Geometry check sheet. Reference: the model listing, model coordinates, mm. A direction names the side the tool comes from. Round coordinates to 2 decimals unless told otherwise and drop trailing zeros. Write each loop counter-clockwise with the first axis right and the second up, starting at its lowest first coordinate (ties: lowest second). Pieces come first, ordered by that corner, then holes. Notation, with made-up numbers: M 32.25,45.5 L 76.25,45.5 A34 ccw 76.25,81.5 Z; hole C 75,-12 d5. An arc over 180 degrees is marked long. One line per item, written item: value. Start each with the question number.
1. Section check D-D (x = 1.75). Count the separate pieces of the cut face and the enclosed holes in it, and give its area (3 significant figures).
2. Access from +Z, -Z, +X, -X, +Y, -Y to the whole of each face (thin tool, end or side, straight path). Record for faces 4 (the cylindrical face through (-10.5, 3.5, 0)), 5 (the flat face through (0, 3, -15)), 6 (the flat face through (7.5, 10, -19)), 7 (the flat face through (5, 15, -15)), 8 (the flat face through (-7.5, 10, -19)).
3. Section check C-C (z = -18.5). Record the boundary of the cut face in (x, y).
4. Release check for a two-part mould opening along Y. For faces 1 (the flat face through (3, 7, -3)), 2 (the flat face through (-0.5, 4, 9)), 3 (the cylindrical face through (2.72, 4.22, 18.77)) record: pulls with the +Y half, pulls with the -Y half, needs draft (parallel to the pull), parting line crosses it, or undercut.
5. Section check A-A (x = 6.5). Record the boundary of the cut face in (y, z).
6. Section check B-B (y = 15). Record the boundary of the cut face in (x, z), and give its area (3 significant figures).
7. Scan lines: probe 1 along Y at (x, z) = (-4.6, -18.5); probe 2 along X at (y, z) = (3, -16); probe 3 along Y at (x, z) = (-1.55, 16.5). Record each from-to range of solid material in increasing order. Write a range as [from, to].
8. Depth check by flat-ended pin: P1, Ø3.5, axis at y = 3.5, z = 16, coming from the -X side; P2, Ø5.5, axis at y = 3.5, z = 16.5, coming from the +X side; P3, Ø5.5, axis at x = 5, y = 16, coming from the +Z side; P4, Ø4, axis at y = 5, z = -18.5, coming from the +X side. Enter the tip coordinate at first touch or a pass-through.
from build123d import *

# Parameters (mm, degrees)
SKETCH1_W           = 5
SKETCH1_H           = 7
BOSS_EXTRUDE1_DEPTH = 7
SKETCH3_R           = 2.38125
CUT_EXTRUDE2_DEPTH  = 29.969811874
FILLET2_R           = 3.5
SKETCH5_W           = 1
SKETCH5_H           = 8.5
CUT_EXTRUDE4_DEPTH  = 27.253571186
SKETCH6_R           = 1.5
CUT_EXTRUDE5_DEPTH  = 27.253571186
SKETCH8_W           = 5
SKETCH8_H           = 7
BOSS_EXTRUDE2_DEPTH = 13
FILLET3_DEPTH       = 20
FILLET3_2_DEPTH     = 8.22694
FILLET3_START       = -9.48212727
FILLET3_3_DEPTH     = 6.98212727
FILLET3_START_2     = 2.5
FILLET3_4_DEPTH     = 6.98212727
FILLET3_START_3     = 7
FILLET3_5_DEPTH     = 13.0000001
CHAMFER1_SIZE       = 2.5
CHAMFER2_SIZE       = 1
SKETCH9_R           = 1.5
CUT_EXTRUDE7_DEPTH  = 36.832945734


with BuildPart() as part:
    # Sketch1 → Boss-Extrude1 (new body)
    with BuildSketch(Plane(origin=(0, 0, 0), x_dir=(1, 0, 0), z_dir=(0, 1, 0))):
        with BuildLine():
            Line((-5, -5), (-5, -11.456439237))
            ThreePointArc((-5, -11.456439237), (0, -12.5), (5, -11.456439237))
            Line((5, -11.456439237), (5, -5))
            Line((5, -5), (-5, -5))
        make_face()
        with BuildLine():
            ThreePointArc((-11.620226592, 4.606553371), (-11.556942324, -4.763096065), (-5, -11.456439237))
            Line((-5, -11.456439237), (-5, -5))
            Line((-5, -5), (5, -5))
            Line((5, -5), (5, -11.456439237))
            ThreePointArc((5, -11.456439237), (10.458250332, -6.846531969), (12.5, 0))
            ThreePointArc((12.5, 0), (12.27808683, 2.344905926), (11.620226592, 4.606553371))
            ThreePointArc((11.620226592, 4.606553371), (0, 12.5), (-11.620226592, 4.606553371))
        make_face()
        with BuildLine():
            Line((-5, -11.456439237), (-5, -20))
            Line((-5, -20), (5, -20))
            Line((5, -20), (5, -11.456439237))
            ThreePointArc((5, -11.456439237), (0, -12.5), (-5, -11.456439237))
        make_face()
        with BuildLine():
            Line((-7.5, 15), (-11.620226592, 4.606553371))
            ThreePointArc((-11.620226592, 4.606553371), (0, 12.5), (11.620226592, 4.606553371))
            Line((11.620226592, 4.606553371), (7.5, 15))
            Line((7.5, 15), (2.5, 15))
            Line((2.5, 15), (-2.5, 15))
            Line((-2.5, 15), (-7.5, 15))
        make_face()
        with Locations((-5, 18.5)):
            Rectangle(SKETCH1_W, SKETCH1_H)
        with Locations((5, 18.5)):
            Rectangle(SKETCH1_W, SKETCH1_H)
    extrude(amount=BOSS_EXTRUDE1_DEPTH)

    # Sketch3 → Cut-Extrude2 (cut, through all)
    with BuildSketch(Plane.ZY.offset(5)):
        with Locations((16.5, 3.5)):
            Circle(SKETCH3_R)
    extrude(amount=-CUT_EXTRUDE2_DEPTH, mode=Mode.SUBTRACT)

    # Fillet2
    fillet2_edges = [part.edges().sort_by_distance(p)[0] for p in [
        (0, 0, 20),
        (0, 7, 20),
    ]]
    fillet(fillet2_edges, radius=FILLET2_R - 0.0001)  # a hair under: the kernel refuses the full size

    # Sketch5 → Cut-Extrude4 (cut, through all)
    with BuildSketch(Plane(origin=(0, 7, 0), x_dir=(1, 0, 0), z_dir=(0, 1, 0))):
        with BuildLine():
            ThreePointArc((3, 0), (-1.936491673, 2.291287847), (-0.5, -2.958039892))
            Line((-0.5, -2.958039892), (-0.5, 0))
            Line((-0.5, 0), (0.5, 0))
            Line((0.5, 0), (0.5, -2.958039892))
            ThreePointArc((0.5, -2.958039892), (2.291287847, -1.936491673), (3, 0))
        make_face()
        with BuildLine():
            Line((-0.5, 0), (-0.5, -2.958039892))
            ThreePointArc((-0.5, -2.958039892), (0, -3), (0.5, -2.958039892))
            Line((0.5, -2.958039892), (0.5, 0))
            Line((0.5, 0), (-0.5, 0))
        make_face()
        with BuildLine():
            Line((-0.5, -2.958039892), (-0.5, -16.5))
            Line((-0.5, -16.5), (0.5, -16.5))
            Line((0.5, -16.5), (0.5, -2.958039892))
            ThreePointArc((0.5, -2.958039892), (0, -3), (-0.5, -2.958039892))
        make_face()
        with Locations((0, -20.75)):
            Rectangle(SKETCH5_W, SKETCH5_H)
    extrude(amount=-CUT_EXTRUDE4_DEPTH, mode=Mode.SUBTRACT)

    # Sketch6 → Cut-Extrude5 (cut, through all)
    with BuildSketch(Plane(origin=(0, 7, 0), x_dir=(1, 0, 0), z_dir=(0, 1, 0))):
        with Locations(Location((7.5, 0, 0), (0, 0, 270))):
            Circle(SKETCH6_R)
        with BuildLine():
            Line((-9, 1.5), (-6, 1.5))
            ThreePointArc((-6, 1.5), (-4.5, 0), (-6, -1.5))
            Line((-6, -1.5), (-9, -1.5))
            ThreePointArc((-9, -1.5), (-10.5, 0), (-9, 1.5))
        make_face()
    extrude(amount=-CUT_EXTRUDE5_DEPTH, mode=Mode.SUBTRACT)

    # Sketch8 → Boss-Extrude2 (add)
    with BuildSketch(Plane(origin=(0, 7, 0), x_dir=(1, 0, 0), z_dir=(0, 1, 0))):
        with Locations((-5, 18.5)):
            Rectangle(SKETCH8_W, SKETCH8_H)
        with Locations((5, 18.5)):
            Rectangle(SKETCH8_W, SKETCH8_H)
    extrude(amount=BOSS_EXTRUDE2_DEPTH)

    # Fillet3: read off the stored shape, not the designer's step
    # Fillet3 outline → Fillet3 (add)
    with BuildSketch(Plane(origin=(0, 0, 0), x_dir=(1, 0, 0), z_dir=(0, 1, 0))):
        with BuildLine():
            Line((7.5, 15), (7.592033284, 15))
            ThreePointArc((7.592033284, 15), (7.523061504, 15.475245132), (7.5, 15.954915028))
            Line((7.5, 15.954915028), (7.5, 15))
        make_face()
        with BuildLine():
            Line((-7.5, 15), (-7.5, 15.954915028))
            ThreePointArc((-7.5, 15.954915028), (-7.523061504, 15.475245132), (-7.592033284, 15))
            Line((-7.592033284, 15), (-7.5, 15))
        make_face()
    extrude(amount=FILLET3_DEPTH)

    # Fillet3 2 outline → Fillet3 2 (add)
    with BuildSketch(Plane(origin=(0, 0, 0), x_dir=(1, 0, 0), z_dir=(0, 1, 0))):
        with BuildLine():
            Line((7.5, 15), (7.851909363, 14.11229368))
            ThreePointArc((7.851909363, 14.11229368), (7.701399823, 14.550124532), (7.592033284, 15))
            Line((7.592033284, 15), (7.5, 15))
        make_face()
        with BuildLine():
            Line((-7.5, 15), (-7.592033284, 15))
            ThreePointArc((-7.592033284, 15), (-7.701399823, 14.550124532), (-7.851909363, 14.11229368))
            Line((-7.851909363, 14.11229368), (-7.5, 15))
        make_face()
    extrude(amount=FILLET3_2_DEPTH)

    # Fillet3 3 outline → Fillet3 3 (add)
    with BuildSketch(Plane.YZ.offset(FILLET3_START)):
        with BuildLine():
            ThreePointArc((12, -15), (8.464466094, -13.535533906), (7, -10))
            Line((7, -10), (7, -15))
            Line((7, -15), (8.22694, -15))
            Line((8.22694, -15), (12, -15))
        make_face()
    extrude(amount=FILLET3_3_DEPTH)

    # Fillet3 4 outline → Fillet3 4 (add)
    with BuildSketch(Plane.YZ.offset(FILLET3_START_2)):
        with BuildLine():
            ThreePointArc((12, -15), (8.464466094, -13.535533906), (7, -10))
            Line((7, -10), (7, -15))
            Line((7, -15), (8.22694, -15))
            Line((8.22694, -15), (12, -15))
        make_face()
    extrude(amount=FILLET3_4_DEPTH)

    # Fillet3 5 outline → Fillet3 5 (cut)
    with BuildSketch(Plane(origin=(0, 0, 0), x_dir=(1, 0, 0), z_dir=(0, 1, 0)).offset(FILLET3_START_3)):
        with BuildLine():
            ThreePointArc((7.592033284, 15), (7.701399823, 14.550124532), (7.851909363, 14.11229368))
            Line((7.851909363, 14.11229368), (9.482127184, 9.999999966))
            Line((9.482127184, 9.999999966), (9.48212727, 15))
            Line((9.48212727, 15), (7.592033284, 15))
        make_face()
        with BuildLine():
            ThreePointArc((-7.851909363, 14.11229368), (-7.701399823, 14.550124532), (-7.592033284, 15))
            Line((-7.592033284, 15), (-9.48212727, 15))
            Line((-9.48212727, 15), (-9.48212727, 10))
            Line((-9.48212727, 10), (-7.851909363, 14.11229368))
        make_face()
    extrude(amount=FILLET3_5_DEPTH, mode=Mode.SUBTRACT)

    # Chamfer1
    chamfer1_edges = [part.edges().sort_by_distance(p)[0] for p in [
        (-5, 0, -22),
        (5, 0, -22),
    ]]
    chamfer(chamfer1_edges, length=CHAMFER1_SIZE)

    # Chamfer2
    chamfer2_edges = [part.edges().sort_by_distance(p)[0] for p in [
        (-5.046016642, 20, -15),
        (5.046016642, 20, -15),
        (5, 20, -22),
        (-5, 20, -22),
    ]]
    chamfer(chamfer2_edges, length=CHAMFER2_SIZE)

    # Sketch9 → Cut-Extrude7 (cut, through all)
    with BuildSketch(Plane.ZY.offset(7.5)):
        with Locations((-18.5, 15)):
            Circle(SKETCH9_R)
        with Locations((-18.5, 5)):
            Circle(SKETCH9_R)
    extrude(amount=-CUT_EXTRUDE7_DEPTH, mode=Mode.SUBTRACT)


solid = part.part
Result sheet:
1. separate pieces: 2
1. enclosed holes: 1
1. area: 188 mm2
2. face 4: +Y, -Y
2. face 5: -Z, +Y, -Y
2. face 6: -Z, +X, +Y, -Y
2. face 7: +Z, +X, -X, +Y
2. face 8: -Z, -X, +Y, -Y
3. outline: M -7.5,0 L -2.5,0 L -2.5,3.5 L -7.5,3.5 Z; M -7.5,6.5 L -2.5,6.5 L -2.5,13.5 L -7.5,13.5 Z; M -7.5,16.5 L -2.5,16.5 L -2.5,20 L -7.5,20 Z; M 2.5,0 L 7.5,0 L 7.5,3.5 L 2.5,3.5 Z; M 2.5,6.5 L 7.5,6.5 L 7.5,13.5 L 2.5,13.5 Z; M 2.5,16.5 L 7.5,16.5 L 7.5,20 L 2.5,20 Z
4. face 1: pulls with the +Y half
4. face 2: needs draft
4. face 3: undercut
5. outline: M 0,-19.5 L 2.5,-22 L 19,-22 L 20,-21 L 20,-16 L 19,-15 L 12,-15 A5 cw 7,-10 L 7,-1.12 L 0,-1.12 Z; M 0,1.12 L 7,1.12 L 7,10.68 L 0,10.68 Z; hole C 5,-18.5 d3; hole C 15,-18.5 d3
6. outline: M -7.59,-15 A5 cw -7.5,-15.95 L -7.5,-17 L -2.5,-17 L -2.5,-15 Z; M -7.5,-22 L -2.5,-22 L -2.5,-20 L -7.5,-20 Z; M 2.5,-22 L 7.5,-22 L 7.5,-20 L 2.5,-20 Z; M 2.5,-17 L 7.5,-17 L 7.5,-15.95 A5 cw 7.59,-15 L 2.5,-15 Z
6. area: 40.1 mm2
7. probe 1: y = [0, 3.5], [6.5, 13.5], [16.5, 20]
7. probe 2: x = [-7.5, -2.5], [2.5, 7.5]
7. probe 3: y = [0, 1.12], [5.88, 7]
8. P1: passes through
8. P2: stops at x = 5
8. P3: stops at z = -15
8. P4: stops at x = 7.5
